CAD build for the part. Positions are in the model's coordinates, mm. A direction names the side the tool comes from. Give positions to 0.01 mm unless a question says otherwise; leave off trailing zeros. Write each loop counter-clockwise with the first axis right and the second up, starting at its lowest first coordinate (ties: lowest second). Pieces come first, ordered by that corner, then holes. Notation, with made-up numbers: (16, 53) - (73, 53) arc R20 cw to (73, 62) - close; hole circle Ø10 at (8, 64). An arc over 180 degrees is marked (long way). Put each result on its own line as item: value. Start each with the question number.
1. Drop flat-ended pins along their axis: pin 1 (1 mm diameter, centred on x = 3, y = -21, fed in from -Z); pin 2 (2 mm diameter, centred on y = 20.5, z = 2, fed in from -X); pin 3 (3.5 mm diameter, centred on x = 0, z = 0, fed in from +Y). Give the stop position or say it passes through.
2. Mould opens along Y. For faces 5 (the flat face through (-1, -4.52, -3)), 6 (the flat face through (0, -25, 3.5)), 7 (the cylindrical face through (-0.521, -16.931, -3.966)), 8 (the conical face through (0.35, 25.96, -0.11)) say: +Y half, -Y half, draft (parallel to the pull), parting line (faces both ways), or undercut.
3. Cut at A-A on y = 13. List the corners of the cut face in (x, z).
4. Wall check: line 1 (Y direction, x = 3.5, z = 1); line 2 (Z direction, x = 0, y = 33.25); line 3 (Z direction, x = 3.25, y = -31). Give the ranges that are in metal, low to high.
5. Tool access for faces 1 (the flat face through (1.8, 35, 1.4)), 2 (the cylindrical face through (-2.003, 30.944, -0.631)), 3 (the flat face through (0, 31, 3.5)), 4 (the cylindrical face through (-3, -4, 0)): list every direction of +Z, -Z, +X, -X, +Y, -Y with a clear straight run to the whole face (end or side of a thin tool).
from build123d import *

# Parameters (mm, degrees)
CORTAR_EXTRUIR1_DEPTH         = 36.454195802
CORTAR_EXTRUIR1_DEPTH_BACK    = 36.454195802
CROQUIS2_W                    = 0.5
CROQUIS2_H                    = 8
CROQUIS2_H_2                  = 7
TALADRO_ROSCADO_M5X0_81_D     = 4.2
TALADRO_ROSCADO_M5X0_81_DEPTH = 8
TALADRO_ROSCADO_M5X0_81_TIP   = 1.2618073


with BuildPart() as part:
    # Croquis1 → Revolución1 (revolve)
    with BuildSketch(Plane.XY):
        Polygon((0, 35), (4, 35), (4, -3.52), (3, -3.52), (3, -4.52), (4, -4.52), (4, -29), (3, -29), (3, -30), (4, -30), (4, -35), (0, -35), align=None)
    revolve(axis=Axis((0, -35, 0), (0, 1, 0)))

    # Croquis2 → Cortar-Extruir1 (cut, two sides: drawn at the far end of the back side and taken through both)
    with BuildSketch(Plane(origin=(0, 0, 0), x_dir=(0, 0, -1), z_dir=(1, 0, 0)).offset(-CORTAR_EXTRUIR1_DEPTH_BACK)):
        with Locations((-3.75, -25)):
            Rectangle(CROQUIS2_W, CROQUIS2_H)
        with Locations((-3.75, 31.5)):
            Rectangle(CROQUIS2_W, CROQUIS2_H_2)
    extrude(amount=CORTAR_EXTRUIR1_DEPTH + CORTAR_EXTRUIR1_DEPTH_BACK, mode=Mode.SUBTRACT)

    # Taladro roscado M5x0.81
    with Locations(Plane(origin=(0, 35, 0), x_dir=(1, 0, 0), z_dir=(0, 1, 0))):
        with Locations((0, 0)):
            Hole(TALADRO_ROSCADO_M5X0_81_D / 2, depth=TALADRO_ROSCADO_M5X0_81_DEPTH)
            with Locations((0, 0, -(TALADRO_ROSCADO_M5X0_81_DEPTH + TALADRO_ROSCADO_M5X0_81_TIP / 2))):  # 118° drill point
                Cone(0, TALADRO_ROSCADO_M5X0_81_D / 2, TALADRO_ROSCADO_M5X0_81_TIP, mode=Mode.SUBTRACT)


solid = part.part
Report:
1. pin 1: stops at z = -3.12
1. pin 2: stops at x = -3.87
1. pin 3: stops at y = 26.79
2. face 5: undercut
2. face 6: undercut
2. face 7: draft
2. face 8: +Y half
3. outline: circle Ø8 at (0, 0)
4. line 1: y = -35 to -30, -29 to -4.52, -3.52 to 35
4. line 2: z = -4 to -2.1, 2.1 to 3.5
4. line 3: z = -2.33 to 2.33
5. face 1: +Z, -Z, +X, -X, +Y
5. face 2: +Y
5. face 3: +Z, +X, -X, +Y
5. face 4: none
